from build123d import *

# Parameters (mm, degrees)
F0_W           = 127
F0_H           = 101.6
F1_DEPTH       = 38.1
F2_W           = 76.2
F2_H           = 50.8
F3_DEPTH       = 9.525
F4_R           = 6.35
F6_D           = 6.35
F6_CBORE_D     = 12.7
F6_CBORE_DEPTH = 6.35
F7_W           = 3.175
F7_H           = 22.225
F8_DEPTH       = 127.001
F10_D          = 5.1054
F10_DEPTH      = 19.05
F10_TIP        = 1.5338169022
F11_W          = 12.7
F11_H          = 38.1
F12_DEPTH      = 12.7
F13_R          = 7.9375
F15_DEPTH      = 3.175
F16_W          = 57.15
F16_H          = 31.75
F17_DEPTH      = 6.35
F18_R          = 6.35
F20_D          = 3.175
F20_DEPTH      = 9.525
F20_TIP        = 0.9538662327
F21_W          = 44.45
F21_H          = 76.2
F22_DEPTH      = 2.38125
F23_R          = 6.35


# Not quite as in the source:
# - a feature of the source that left no trace in its solid (it failed there, or was rolled back) is left out


with BuildPart() as f1:
    # F0 (on Top) → F1 (new body)
    with BuildSketch(Plane.XY):
        Rectangle(F0_W, F0_H)
    extrude(amount=F1_DEPTH)

    # F2 (on face) → F3 (cut)
    with BuildSketch(Plane.XY.offset(38.1)):
        Rectangle(F2_W, F2_H)
    extrude(amount=-F3_DEPTH, mode=Mode.SUBTRACT)

    # F4
    f4_edges = [f1.edges().sort_by_distance(p)[0] for p in [
        (-38.1, 25.4, 33.3375),
        (38.1, 25.4, 33.3375),
        (38.1, -25.4, 33.3375),
        (-38.1, -25.4, 33.3375),
    ]]
    fillet(f4_edges, radius=F4_R)

    # F6 (through all)
    with Locations(Plane.XY.offset(38.1)):
        with Locations((-50.8, 38.1), (50.8, 38.1), (50.8, -38.1), (-50.8, -38.1)):
            CounterBoreHole(F6_D / 2, F6_CBORE_D / 2, F6_CBORE_DEPTH)

    # F7 (on face) → F8 (cut, through all)
    with BuildSketch(Plane.YZ.offset(63.5)):
        with Locations((-49.2125, 17.4625)):
            Rectangle(F7_W, F7_H)
        with Locations((49.2125, 17.4625)):
            Rectangle(F7_W, F7_H)
    extrude(amount=-F8_DEPTH, mode=Mode.SUBTRACT)

    # F10
    with Locations(Plane.XY.offset(28.575)):
        with Locations((-31.75, 19.05), (-31.75, -19.05), (31.75, -19.05), (31.75, 19.05)):
            Hole(F10_D / 2, depth=F10_DEPTH)
            with Locations((0, 0, -(F10_DEPTH + F10_TIP / 2))):  # 118° drill point
                Cone(0, F10_D / 2, F10_TIP, mode=Mode.SUBTRACT)

    # F11 (on face) → F12 (cut)
    with BuildSketch(Plane.XY.offset(38.1)):
        with Locations((-57.15, 0)):
            Rectangle(F11_W, F11_H)
        with Locations((57.15, 0)):
            Rectangle(F11_W, F11_H)
    extrude(amount=-F12_DEPTH, mode=Mode.SUBTRACT)

    # F13
    f13_edges = [f1.edges().sort_by_distance(p)[0] for p in [
        (-50.8, 19.05, 31.75),
        (-50.8, -19.05, 31.75),
        (50.8, 19.05, 31.75),
        (50.8, -19.05, 31.75),
    ]]
    fillet(f13_edges, radius=F13_R)

    # F14 (on face) → F15 (cut)
    with BuildSketch(Plane(origin=(0, 0, 0), x_dir=(1, 0, 0), z_dir=(0, 0, -1))):
        with BuildLine():
            Line((-31.75, -25.4), (31.75, -25.4))
            ThreePointArc((31.75, -25.4), (36.2401280605, -23.5401280605), (38.1, -19.05))
            Line((38.1, -19.05), (38.1, 19.05))
            ThreePointArc((38.1, 19.05), (36.2401280605, 23.5401280605), (31.75, 25.4))
            Line((31.75, 25.4), (-31.75, 25.4))
            ThreePointArc((-31.75, 25.4), (-36.2401280605, 23.5401280605), (-38.1, 19.05))
            Line((-38.1, 19.05), (-38.1, -19.05))
            ThreePointArc((-38.1, -19.05), (-36.2401280605, -23.5401280605), (-31.75, -25.4))
        make_face()
    extrude(amount=-F15_DEPTH, mode=Mode.SUBTRACT)

    # F16 (on face) → F17 (cut)
    with BuildSketch(Plane(origin=(0, 0, 3.175), x_dir=(1, 0, 0), z_dir=(0, 0, -1))):
        Rectangle(F16_W, F16_H)
    extrude(amount=-F17_DEPTH, mode=Mode.SUBTRACT)

    # F18
    f18_edges = [f1.edges().sort_by_distance(p)[0] for p in [
        (-28.575, -15.875, 6.35),
        (-28.575, 15.875, 6.35),
        (28.575, -15.875, 6.35),
        (28.575, 15.875, 6.35),
    ]]
    fillet(f18_edges, radius=F18_R)

    # F20
    with Locations(Plane.XY.offset(38.1)):
        with Locations((-25.4, 42.8625), (25.4, 42.8625), (-25.4, -42.8625), (25.4, -42.8625)):
            Hole(F20_D / 2, depth=F20_DEPTH)
            with Locations((0, 0, -(F20_DEPTH + F20_TIP / 2))):  # 118° drill point
                Cone(0, F20_D / 2, F20_TIP, mode=Mode.SUBTRACT)

    # F21 (on face) → F22 (cut)
    with BuildSketch(Plane.XY.offset(38.1)):
        Rectangle(F21_W, F21_H)
    extrude(amount=-F22_DEPTH, mode=Mode.SUBTRACT)

    # F23
    f23_edges = [f1.edges().sort_by_distance(p)[0] for p in [
        (-22.225, 38.1, 36.909375),
        (22.225, 38.1, 36.909375),
        (22.225, -38.1, 36.909375),
        (-22.225, -38.1, 36.909375),
    ]]
    fillet(f23_edges, radius=F23_R)


solid = f1.part
Input: part model. Units: mm. Frame: model coordinates. A direction names the side the tool comes from. Give positions to 0.01 mm unless a question says otherwise; leave off trailing zeros. Order: outer loops, then holes, each group sorted by start corner. A loop starts at its lowest first (then second) coordinate and runs counter-clockwise, first axis right, second up. Notation, with made-up numbers: M 14.25,5 L 45.25,5 A20 cw 45.25,27 Z; hole C 13,-5.75 d6. An arc over 180 degrees is marked long. Answer as a JSON object with one key per item and string values.
1. Cut plane A-A, the plane z = 21. State how many separate pieces and enclosed holes the cut face has, and give its area (3 significant figures).
Result sheet:
{"separate pieces": "1", "enclosed holes": "8", "area": "11,900 mm²"}
2. Cut plane B-B, the plane y = -1. Output: boundary loops of the cut face in (x, z) (3 decimals), and give its area (3 significant figures).
Result sheet:
{"outline": "M -63.5,0 L -38.1,0 L -38.1,3.175 L -28.575,3.175 L -28.575,9.525 L 28.575,9.525 L 28.575,3.175 L 38.1,3.175 L 38.1,0 L 63.5,0 L 63.5,25.4 L 50.8,25.4 L 50.8,38.1 L 38.1,38.1 L 38.1,28.575 L -38.1,28.575 L -38.1,38.1 L -50.8,38.1 L -50.8,25.4 L -63.5,25.4 Z", "area": "3,190 mm²"}
3. Pull-direction query (X, two-part tool) for faces 3 (the flat face through (-61, -19.05, 32)), 4 (the cylindrical face through (-53.83, -37.15, 15.65)), 5 (the cylindrical face through (-53.2, -16.8, 31.7)); classes: +X half, -X half, draft (parallel to the pull), parting line (faces both ways), or undercut.
Result sheet:
{"face 3": "draft", "face 4": "undercut", "face 5": "-X half"}
4. First-contact query: P1, Ø12, axis at x = -22.5, y = 11.5, coming from the -Z side (3 decimals); P2, Ø3, axis at x = 3, z = 22.5, coming from the -Y side (3 decimals); P3, Ø4, axis at x = 53, y = 36, coming from the +Z side. Flat tips, straight axial feed; report the tip coordinate or a pass-through.
Result sheet:
{"P1": "z = 3.175", "P2": "y = -47.625", "P3": "z = 31.75"}
5. Reachability of faces 1 (the flat face through (-54, 37, 31.75)), 2 (the flat face through (0, -25.4, 2)) from +Z, -Z, +X, -X, +Y, -Y: full face, straight path, thin tool, end or side. Return the list, or none.
Result sheet:
{"face 1": "+Z", "face 2": "-Z"}
6. Ray query, line 1 (X direction, y = 19, z = 21); line 2 (X direction, y = 38, z = 33); line 3 (Y direction, x = -3, z = 3). Return the intervals inside material, ascending. Write a range as [from, to].
Result sheet:
{"line 1": "[-63.5, -34.3], [-29.2, 29.2], [34.3, 63.5]", "line 2": "[-63.5, -57.15], [-44.45, 44.45], [57.15, 63.5]", "line 3": "[-50.8, -25.4], [25.4, 50.8]"}
7. Cut plane D-D, the plane x = 42. Output: boundary loops of the cut face in (y, z) (3 decimals), and give its area (3 significant figures).
Result sheet:
{"outline": "M -50.8,0 L 50.8,0 L 50.8,6.35 L 47.625,6.35 L 47.625,28.575 L 50.8,28.575 L 50.8,38.1 L -50.8,38.1 L -50.8,28.575 L -47.625,28.575 L -47.625,6.35 L -50.8,6.35 Z", "area": "3,730 mm²"}
8. Cut plane C-C, the plane x = -8.5. Output: boundary loops of the cut face in (y, z) (3 decimals).
Result sheet:
{"outline": "M -50.8,0 L -25.4,0 L -25.4,3.175 L -15.875,3.175 L -15.875,9.525 L 15.875,9.525 L 15.875,3.175 L 25.4,3.175 L 25.4,0 L 50.8,0 L 50.8,6.35 L 47.625,6.35 L 47.625,28.575 L 50.8,28.575 L 50.8,38.1 L 38.1,38.1 L 38.1,35.719 L 25.4,35.719 L 25.4,28.575 L -25.4,28.575 L -25.4,35.719 L -38.1,35.719 L -38.1,38.1 L -50.8,38.1 L -50.8,28.575 L -47.625,28.575 L -47.625,6.35 L -50.8,6.35 Z"}
